Verification items for the finished model (mm, model axes). A direction names the side the tool comes from. Coordinates: 2 decimals unless noted, no trailing zeros. Order: outer loops, then holes, each group sorted by start corner. A loop starts at its lowest first (then second) coordinate and runs counter-clockwise, first axis right, second up. Notation, with made-up numbers: M 83,-26 L 123,-26 A35 ccw 123,6 Z; hole C 1.5,17 d8. An arc over 180 degrees is marked long. Return JSON: item names as keys, results as strings. Group by question number.
Q1. Thickness scan on probe 1 along X at (y, z) = (19.5, 3.5); probe 2 along Z at (x, y) = (4.5, 34). Record the ranges inside material, lowest first.
Q2. Section check A-A, the plane z = -5. Enter the section's corners in (x, y), then the cut area to 3 significant figures.
Q3. Section check B-B, the plane y = -18. Enter the section's corners in (x, z), then the cut area to 3 significant figures.
Q4. Mould release check, pull along X, two halves, no side actions. Record for faces 3 (the face through (-13.328, -1, 9)), 4 (the face through (19, 1, 30.48)), 5 (the face through (25.4, -1, 2)), 6 (the face through (0, 1, -12.7)): pulls with the +X half, pulls with the -X half, needs draft (parallel to the pull), parting line crosses it, or undercut.
Q5. Go/stop test with a flat-tipped pin: pin 1 Ø1 at (x, y) = (0.5, 13.5) entering from +Z. Record where the tip stops, or that it passes through.
Q6. Access from +Z, -Z, +X, -X, +Y, -Y to the whole of each face (thin tool, end or side, straight path). Record for faces 1 (the face through (13.328, -1, 9)), 2 (the face through (0, 50.8, -16)).
Q7. Section check C-C, the plane x = 3. Enter the section's corners in (y, z), then the cut area to 3 significant figures.
from build123d import *

# Parameters (mm, degrees)
F0_W     = 50.8
F0_H     = 101.6
F1_DEPTH = 25.4
F2_W     = 26.6550015658
F2_H     = 101.6
F3_DEPTH = 38.1
F4_DEPTH = 25.4
F5_DEPTH = 25.4
F6_DEPTH = 20.32


with BuildPart() as f1:
    # F0 (on Top) → F1 (new body, symmetric)
    with BuildSketch(Plane.XY):
        Rectangle(F0_W, F0_H)
    extrude(amount=F1_DEPTH, both=True)

    # F2 (on face) → F3 (cut)
    with BuildSketch(Plane.XY.offset(25.4)):
        Rectangle(F2_W, F2_H)
    extrude(amount=-F3_DEPTH, mode=Mode.SUBTRACT)

    # F4 (add): a face of the model
    f4_faces = [f1.faces().sort_by_distance(p)[0] for p in [
        (-19.3637503915, 0, 25.4),
    ]]
    extrude(f4_faces, amount=F4_DEPTH)

    # F5 (add): a face of the model
    f5_faces = [f1.faces().sort_by_distance(p)[0] for p in [
        (19.3637503915, 0, 25.4),
    ]]
    extrude(f5_faces, amount=F5_DEPTH)

    # F6 (cut): faces of the model
    f6_faces = [f1.faces().sort_by_distance(p)[0] for p in [
        (19.3637503915, 0, 50.8),
        (-19.3637503915, 0, 50.8),
    ]]
    extrude(f6_faces, amount=-F6_DEPTH, mode=Mode.SUBTRACT)


solid = f1.part
Numbers:
{
 "1": {"probe 1": "x = -25.4 to -13.33, 13.33 to 25.4", "probe 2": "z = -25.4 to -12.7"},
 "2": {"outline": "M -25.4,-50.8 L -13.33,-50.8 L -13.33,50.8 L -25.4,50.8 Z; M 13.33,-50.8 L 25.4,-50.8 L 25.4,50.8 L 13.33,50.8 Z", "area": "2,450 mm2"},
 "3": {"outline": "M -25.4,-25.4 L 25.4,-25.4 L 25.4,30.48 L 13.33,30.48 L 13.33,-12.7 L -13.33,-12.7 L -13.33,30.48 L -25.4,30.48 Z", "area": "1,690 mm2"},
 "4": {"face 3": "undercut", "face 4": "needs draft", "face 5": "pulls with the +X half", "face 6": "undercut"},
 "5": {"pin 1": "stops at z = -12.7"},
 "6": {"face 1": "+Z, +Y, -Y", "face 2": "+Z, -Z, +X, -X, +Y"},
 "7": {"outline": "M -50.8,-25.4 L 50.8,-25.4 L 50.8,-12.7 L -50.8,-12.7 Z", "area": "1,290 mm2"}
}
